Source: CAD feature listing. Evaluate the final solid. Frame: model axes, mm. Face numbers are marked on the shaded views. A direction names the side the tool comes from. Coordinates: 2 decimals unless noted, no trailing zeros. Order: outer loops, then holes, each group sorted by start corner. A loop starts at its lowest first (then second) coordinate and runs counter-clockwise, first axis right, second up. Notation, with made-up numbers: (41, 2) - (74, 2) arc R13 cw to (74, 24) - close; hole circle Ø2 at (44, 68.25). An arc over 180 degrees is marked (long way). One line per question, with ' | ' between items.
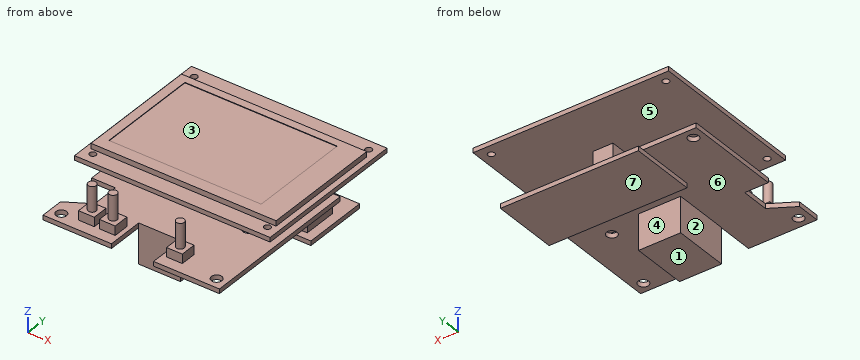
Autodesk Inventor part; units mm, degrees
ref_plane "YZ Plane" through (0, 0, 0) normal (1, 0, 0) x (0, 1, 0)
ref_plane "XZ Plane" through (0, 0, 0) normal (0, 1, 0) x (-1, 0, 0)
ref_plane "XY Plane" through (0, 0, 0) normal (0, 0, 1) x (1, 0, 0)
sketch "Umriss_Sensorplatine" plane through (0, 0, 0) normal (0, 0, 1) x (1, 0, 0)
  line L0 (0, 62) -> (67, 62)
  line L1 (67, 62) -> (67, 0)
  line L2 (67, 0) -> (42, 0)
  line L3 (42, 0) -> (42, 14)
  line L4 (42, 14) -> (26, 14)
  line L5 (26, 14) -> (26, 0)
  line L6 (26, 0) -> (0, 0)
  line L7 (9, 14.3) -> (9, 25)
  line L8 (9, 25) -> (0, 25)
  line L9 (0, 0) -> (0, 9)
  line L10 (0, 25) -> (0, 62)
  circle A0 centre (63, 4) radius 2
  circle A1 centre (4, 4) radius 2
  circle A2 centre (55, 31) radius 2
  circle A3 centre (4, 58) radius 2
  line L11 (4, 4) -> (63, 4) construction
  line L12 (4, 4) -> (4, 58) construction
  line L13 (0, 9) -> (9, 14.3)
  dimension "d0" = 4
  dimension "d2" = 4
  dimension "d3" = 4
  dimension "d4" = 4
  dimension "d5" = 67
  dimension "d6" = 26
  dimension "d7" = 42
  dimension "d8" = 14
  dimension "d9" = 4
  dimension "d11" = 25
  dimension "d12" = 9
  dimension "d13" = 62
  dimension "d14" = 31
  dimension "d15" = 55
  dimension "d67" = 14.3
  dimension "d68" = 9
extrude "Sensorplatine" add sketch "Umriss_Sensorplatine" along normal blind 1.75
sketch "Tasterprojektion" plane through (0, 0, 1.75) normal (0, 0, 1) x (1, 0, 0)
  line L0 (0, 0) -> (26, 0) construction
  line L1 (26, 0) -> (26, 14) construction
  line L2 (26, 14) -> (42, 14) construction
  line L3 (42, 14) -> (42, 0) construction
  line L4 (42, 0) -> (67, 0) construction
  line L5 (67, 0) -> (67, 62) construction
  line L6 (67, 62) -> (0, 62) construction
  line L7 (0, 62) -> (0, 25) construction
  line L8 (0, 9) -> (0, 0) construction
  line L9 (0, 7.3) -> (67, 7.3) construction
  circle A0 centre (13.3, 7.3) radius 1.525
  circle A1 centre (21.25, 7.3) radius 1.525
  circle A2 centre (46.75, 7.3) radius 1.525
  line L10 (43.75, 10.3) -> (49.75, 10.3)
  line L11 (49.75, 10.3) -> (49.75, 4.3)
  line L12 (49.75, 4.3) -> (43.75, 4.3)
  line L13 (43.75, 4.3) -> (43.75, 10.3)
  line L14 (43.75, 10.3) -> (49.75, 4.3) construction
  line L15 (49.75, 10.3) -> (43.75, 4.3) construction
  line L16 (18.25, 10.3) -> (24.25, 10.3)
  line L17 (24.25, 10.3) -> (24.25, 4.3)
  line L18 (24.25, 4.3) -> (18.25, 4.3)
  line L19 (18.25, 4.3) -> (18.25, 10.3)
  line L20 (18.25, 10.3) -> (24.25, 4.3) construction
  line L21 (24.25, 10.3) -> (18.25, 4.3) construction
  line L22 (10.3, 10.3) -> (16.3, 10.3)
  line L23 (16.3, 10.3) -> (16.3, 4.3)
  line L24 (16.3, 4.3) -> (10.3, 4.3)
  line L25 (10.3, 4.3) -> (10.3, 10.3)
  line L26 (10.3, 10.3) -> (16.3, 4.3) construction
  line L27 (16.3, 10.3) -> (10.3, 4.3) construction
  dimension "d19" = 7.3
  dimension "d20" = 3.05
  dimension "d21" = 13.3
  dimension "d22" = 21.25
  dimension "d23" = 46.75
  dimension "d24" = 6
  dimension "d25" = 6
extrude "Grundkoerper Taster" add sketch "Tasterprojektion" along normal blind 3.5
extrude "Nubsis Taster" add sketch "Tasterprojektion" along normal blind 13 contours A0 | A1 | A2
sketch "Sketch3" plane through (0, 0, 1.75) normal (0, 0, 1) x (1, 0, 0)
  line L0 (37.3343, 37.5267) -> (44.9961, 37.5267)
  line L1 (44.9961, 37.5267) -> (44.9961, 54.2692)
  line L2 (44.9961, 54.2692) -> (37.3343, 54.2692)
  line L3 (37.3343, 54.2692) -> (37.3343, 37.5267)
  line L4 (37.3343, 37.5267) -> (44.9961, 54.2692) construction
  line L5 (44.9961, 37.5267) -> (37.3343, 54.2692) construction
  point P0 (41.1652, 45.898)
extrude "Steckverbinder" add sketch "Sketch3" along normal blind 12
sketch "Sketch4" plane through (0, 0, 13.75) normal (0, 0, 1) x (1, 0, 0)
  line L0 (0, 62) -> (0, 25) construction
  line L1 (0, 25) -> (9, 25) construction
  line L2 (37.3343, 37.5267) -> (37.3343, 54.2692) construction
  line L3 (37.3343, 54.2692) -> (44.9961, 54.2692) construction
  line L4 (44.9961, 54.2692) -> (44.9961, 37.5267) construction
  line L5 (44.9961, 37.5267) -> (37.3343, 37.5267) construction
  line L6 (0, 0) -> (26, 0) construction
  line L7 (26, 0) -> (26, 14) construction
  line L8 (26, 14) -> (42, 14) construction
  line L9 (42, 14) -> (42, 0) construction
  line L10 (42, 0) -> (67, 0) construction
  line L11 (67, 0) -> (67, 62) construction
  line L12 (67, 62) -> (0, 62) construction
  line L13 (0, 62) -> (0, 25) construction
  line L14 (0, 25) -> (9, 25) construction
  line L15 (9, 25) -> (9, 14.3) construction
  line L16 (0, 9) -> (0, 0) construction
  circle A0 centre (63, 4) radius 2 construction
  circle A1 centre (4, 4) radius 2 construction
  circle A2 centre (55, 31) radius 2 construction
  circle A3 centre (4, 58) radius 2 construction
  line L17 (24.25, 10.3) -> (24.25, 4.3) construction
  line L18 (24.25, 4.3) -> (18.25, 4.3) construction
  line L19 (18.25, 4.3) -> (18.25, 10.3) construction
  line L20 (18.25, 10.3) -> (24.25, 10.3) construction
  line L21 (49.75, 10.3) -> (49.75, 4.3) construction
  line L22 (49.75, 4.3) -> (43.75, 4.3) construction
  line L23 (43.75, 4.3) -> (43.75, 10.3) construction
  line L24 (43.75, 10.3) -> (49.75, 10.3) construction
  line L25 (16.3, 10.3) -> (16.3, 4.3) construction
  line L26 (16.3, 4.3) -> (10.3, 4.3) construction
  line L27 (10.3, 4.3) -> (10.3, 10.3) construction
  line L28 (10.3, 10.3) -> (16.3, 10.3) construction
  line L29 (0.5, 15.5) -> (74.8, 15.5)
  line L30 (74.8, 15.5) -> (74.8, 75.5)
  line L31 (74.8, 75.5) -> (0.5, 75.5)
  line L32 (0.5, 75.5) -> (0.5, 15.5)
  line L33 (4.5, 19.5) -> (70.8, 19.5) construction
  line L34 (70.8, 19.5) -> (70.8, 71.5) construction
  line L35 (70.8, 71.5) -> (4.5, 71.5) construction
  line L36 (4.5, 71.5) -> (4.5, 19.5) construction
  circle A4 centre (70.8, 71.5) radius 1.25
  circle A5 centre (4.5, 71.5) radius 1.25
  circle A6 centre (4.5, 19.5) radius 1.25
  circle A7 centre (70.8, 19.5) radius 1.25
  line L37 (9, 14.3) -> (0, 9)
  dimension "d32" = 0.5
  dimension "d33" = 74.3
  dimension "d34" = 60
  dimension "d35" = 4
  dimension "d36" = 4
  dimension "d37" = 4
  dimension "d38" = 4
  dimension "d39" = 2.5
  dimension "d70" = 13.5
  dimension "d71" = 66.3
  dimension "d72" = 52
  dimension "d73" = 62
extrude "Grundplatine Display" add sketch "Sketch4" along normal blind 1.7
sketch "Sketch5" plane through (0, 0, 15.45) normal (0, 0, 1) x (1, 0, 0)
  line L0 (0.5, 15.5) -> (74.8, 15.5)
  line L1 (74.8, 15.5) -> (74.8, 75.5)
  line L2 (0.5, 75.5) -> (0.5, 15.5)
  circle A0 centre (70.8, 19.5) radius 1.25 construction
  circle A1 centre (4.5, 19.5) radius 1.25 construction
  circle A2 centre (4.5, 71.5) radius 1.25 construction
  circle A3 centre (70.8, 71.5) radius 1.25 construction
  line L3 (0.5, 15.5) -> (74.8, 15.5) construction
  line L4 (74.8, 15.5) -> (74.8, 75.5) construction
  line L5 (74.8, 75.5) -> (0.5, 75.5) construction
  line L6 (0.5, 75.5) -> (0.5, 15.5) construction
  line L7 (2.3, 21.5) -> (72.65, 21.5)
  line L8 (72.65, 21.5) -> (72.65, 68)
  line L9 (72.65, 68) -> (2.3, 68)
  line L10 (2.3, 68) -> (2.3, 21.5)
  point P0 (0, 0)
  dimension "d42" = 6
  dimension "d43" = 7.5
  dimension "d44" = 2.15
  dimension "d45" = 1.8
extrude "Glaskoerper Display" add sketch "Sketch5" along normal blind 2
sketch "Display" plane through (0, 0, 17.45) normal (0, 0, 1) x (1, 0, 0)
  line L0 (2.3, 21.5) -> (72.65, 21.5) construction
  line L1 (72.65, 21.5) -> (72.65, 68) construction
  line L2 (72.65, 68) -> (2.3, 68) construction
  line L3 (2.3, 68) -> (2.3, 21.5) construction
  line L4 (5.8, 26) -> (63.65, 26)
  line L5 (63.65, 26) -> (63.65, 65)
  line L6 (63.65, 65) -> (5.8, 65)
  line L7 (5.8, 65) -> (5.8, 26)
  line L8 (11.3777, 48.5369) -> (83.2025, 48.5369) construction
  line L9 (83.2025, 48.5369) -> (83.2025, 36.2483) construction
  line L10 (83.2025, 36.2483) -> (11.3777, 36.2483) construction
  line L11 (11.3777, 36.2483) -> (11.3777, 48.5369) construction
  point P0 (0, 0)
  dimension "d48" = 4.5
  dimension "d49" = 3
  dimension "d50" = 9
  dimension "d51" = 3.5
extrude "Bildausschnitt" cut sketch "Display" against normal blind 0.2
sketch "Sketch7" plane through (0, 0, 0) normal (0, 0, -1) x (-1, 0, 0)
  line L0 (-66, 59.4637) -> (-39.1956, 59.4637)
  line L1 (-39.1956, 59.4637) -> (-39.1956, 46.4689)
  line L2 (-39.1956, 46.4689) -> (-66, 46.4689)
  line L3 (-66, 46.4689) -> (-66, 59.4637)
extrude "Platzhalter_Stiftleiste" add sketch "Sketch7" along normal blind 3.5
sketch "Sketch8" plane through (0, 0, -3.5) normal (0, 0, -1) x (-1, 0, 0)
  line L0 (-39.1956, 59.4637) -> (-39.1956, 46.4689) construction
  line L1 (-39.1956, 46.4689) -> (-66, 46.4689) construction
  line L2 (-66, 46.4689) -> (-66, 59.4637) construction
  line L3 (-66, 59.4637) -> (-39.1956, 59.4637) construction
  circle A0 centre (-4, 58) radius 2 construction
  circle A1 centre (-55, 31) radius 2 construction
  circle A2 centre (-4, 4) radius 2 construction
  circle A3 centre (-63, 4) radius 2 construction
  line L4 (0, 0) -> (-26, 0) construction
  line L5 (0, 9) -> (0, 0) construction
  line L6 (-9, 25) -> (-9, 14.3) construction
  line L7 (0, 25) -> (-9, 25) construction
  line L8 (0, 62) -> (0, 25) construction
  line L9 (-67, 62) -> (0, 62) construction
  line L10 (-67, 0) -> (-67, 62) construction
  line L11 (-42, 0) -> (-67, 0) construction
  line L12 (-42, 14) -> (-42, 0) construction
  line L13 (-26, 14) -> (-42, 14) construction
  line L14 (-26, 0) -> (-26, 14) construction
  line L15 (-69.5, 68.6) -> (-17.1, 68.6)
  line L16 (-17.1, 68.6) -> (-17.1, 43.6)
  line L17 (-17.1, 43.6) -> (-69.5, 43.6)
  line L18 (-69.5, 43.6) -> (-69.5, 68.6)
  line L19 (-9, 14.3) -> (0, 9)
  dimension "d56" = 6.6
  dimension "d57" = 2.5
  dimension "d58" = 25
  dimension "d59" = 52.4
extrude "HexaHorst" add sketch "Sketch8" along normal blind 1.7
sketch "Sketch9" plane through (0, 0, 0) normal (0, 0, -1) x (-1, 0, 0)
  line L0 (-67, 62) -> (0, 62)
  line L1 (-26, 14) -> (-42, 14)
  line L2 (-34, 14) -> (-33.5, 62) construction
  line L3 (-41.8906, 35) -> (-25.8906, 35)
  line L4 (-25.8906, 35) -> (-25.8906, 14)
  line L5 (-25.8906, 14) -> (-41.8906, 14)
  line L6 (-41.8906, 14) -> (-41.8906, 35)
  line L7 (-41.8906, 35) -> (-25.8906, 14) construction
  line L8 (-25.8906, 35) -> (-41.8906, 14) construction
  point P0 (-33.8906, 24.5)
  dimension "d62" = 16
  dimension "d63" = 21
extrude "Extrusion10" add sketch "Sketch9" along normal blind 13.5
properties part number "Mockup_Platinen"
(1) Material intervals for L1, parallel to Z at x = 39, y = 57; L2, parallel to Y at x = 63, z = 0.85; L3, parallel to Y at x = 55, z = 1.35, sorted ascending. Write a range as from..to.
Taken from the geometry:
L1: z = -5.2..-3.5, 0..1.75, 13.75..17.25 | L2: y = 0..2, 6..62 | L3: y = 0..29, 33..62
(2) Cut plane A-A (y = 66). Return the cut outline in (x, z), and give its area (3 significant figures).
Taken from the geometry:
outline: (0.5, 13.75) - (74.8, 13.75) - (74.8, 15.45) - (72.65, 15.45) - (72.65, 17.45) - (2.3, 17.45) - (2.3, 15.45) - (0.5, 15.45) - close; (17.1, -5.2) - (69.5, -5.2) - (69.5, -3.5) - (17.1, -3.5) - close | area: 356 mm²
(3) Set-up query: the marked faces 1, 2 and 3. Return all of +Z, -Z, +X, -X, +Y, -Y with unobstructed straight access to the full face (end or side cutting, diameter ignored); none if empty.
Taken from the geometry:
face 1: -Z, +X, -X, +Y, -Y | face 2: -Z, -X, -Y | face 3: +Z
(4) Cut plane B-B (x = 30). Return the cut outline in (y, z), and give its area (3 significant figures).
Taken from the geometry:
outline: (14, -13.5) - (35, -13.5) - (35, 0) - (62, 0) - (62, 1.75) - (14, 1.75) - close; (15.5, 13.75) - (75.5, 13.75) - (75.5, 15.45) - (68, 15.45) - (68, 17.45) - (65, 17.45) - (65, 17.25) - (26, 17.25) - (26, 17.45) - (21.5, 17.45) - (21.5, 15.45) - (15.5, 15.45) - close; (43.6, -5.2) - (68.6, -5.2) - (68.6, -3.5) - (43.6, -3.5) - close | area: 597 mm²
(5) Pin query (flat end, axial travel): P1, Ø2, axis at x = 62.5, y = 38, coming from the -Z side; P2, Ø1.5, axis at x = 27.5, y = 46, coming from the +Z side; P3, Ø1.6, axis at y = 34.5, z = 16.5, coming from the +X side. Return the tip coordinate at first contact, or that it passes through.
Taken from the geometry:
P1: stops at z = 0 | P2: stops at z = 17.25 | P3: stops at x = 72.65
(6) Pull-direction query (Z, two-part tool) for the marked faces 4, 5, 6 and 7; classes: pulls with the +Z half, pulls with the -Z half, needs draft (parallel to the pull), parting line crosses it, or undercut.
Taken from the geometry:
face 4: needs draft | face 5: undercut | face 6: undercut | face 7: pulls with the -Z half
(7) Cut plane C-C (z = 3.5). Return the cut outline in (x, y).
Taken from the geometry:
outline: (10.3, 4.3) - (16.3, 4.3) - (16.3, 10.3) - (10.3, 10.3) - close; (18.25, 4.3) - (24.25, 4.3) - (24.25, 10.3) - (18.25, 10.3) - close; (37.33, 37.53) - (45, 37.53) - (45, 54.27) - (37.33, 54.27) - close; (43.75, 4.3) - (49.75, 4.3) - (49.75, 10.3) - (43.75, 10.3) - close
